```python
from build123d import *

# Parameters (mm, degrees)
SKETCH1_W           = 25.4
SKETCH1_H           = 25.4
BOSS_EXTRUDE1_DEPTH = 6.35


with BuildPart() as part:
    # Sketch1 → Boss-Extrude1 (new body)
    with BuildSketch(Plane.XY):
        with Locations((38.1, 241.3)):
            Rectangle(SKETCH1_W, SKETCH1_H)
        with Locations((88.9, 241.3)):
            Rectangle(SKETCH1_W, SKETCH1_H)
        with Locations((139.7, 241.3)):
            Rectangle(SKETCH1_W, SKETCH1_H)
        Polygon((0, 228.6), (0, 0), (177.8, 0), (177.8, 228.6), (152.4, 228.6), (127, 228.6), (116.0018, 228.6), (116.0018, 215.9), (117.1448, 215.9), (117.1448, 213.3092), (116.0018, 213.3092), (116.0018, 205.6892), (112.5982, 205.6892), (112.5982, 213.3092), (111.4552, 213.3092), (111.4552, 215.9), (112.5982, 215.9), (112.5982, 228.6), (101.6, 228.6), (76.2, 228.6), (65.2018, 228.6), (65.2018, 215.9), (66.3448, 215.9), (66.3448, 213.3092), (65.2018, 213.3092), (65.2018, 205.6892), (61.7982, 205.6892), (61.7982, 213.3092), (60.6552, 213.3092), (60.6552, 215.9), (61.7982, 215.9), (61.7982, 228.6), (50.8, 228.6), (25.4, 228.6), align=None)
    extrude(amount=BOSS_EXTRUDE1_DEPTH)


solid = part.part
```
The listing builds one solid part. Answer for the finished solid, in the listing's coordinates (mm). A direction names the side the tool comes from. Give positions to 0.01 mm unless a question says otherwise; leave off trailing zeros. Loops run counter-clockwise (first coordinate to the right, second up) from the corner with the lowest first, then second, coordinate; pieces in that order, holes last. Notation, with made-up numbers: M -4.75,-20.5 L 36.25,-20.5 A13 cw 36.25,-7.5 Z; hole C 50.25,71 d11. An arc over 180 degrees is marked long. One line per item, written item: value.
1. For faces 4 (the face through (13, 228.6, 3)), 5 (the face through (71, 228.6, 3)), 6 (the face through (152.4, 241, 3)), determine the directions among +Z, -Z, +X, -X, +Y, -Y from which every point of the face is accessible in a straight line to the end or side of a thin tool.
Found:
face 4: +Z, -Z, -X, +Y
face 5: +Z, -Z, +Y
face 6: +Z, -Z, +X, +Y
2. For a pull along X with two mould halves and no side action, classify faces 1 (the face through (88, 0, 3)), 2 (the face through (0, 116, 3)), 3 (the face through (61.798, 222, 3)) as pulls with the +X half, pulls with the -X half, needs draft (parallel to the pull), parting line crosses it, or undercut.
Found:
face 1: needs draft
face 2: pulls with the -X half
face 3: undercut
3. Section A-A on y = 210 is taken. Determine the outline of the cut face in (x, z).
Found:
outline: M 0,0 L 61.8,0 L 61.8,6.35 L 0,6.35 Z; M 65.2,0 L 112.6,0 L 112.6,6.35 L 65.2,6.35 Z; M 116,0 L 177.8,0 L 177.8,6.35 L 116,6.35 Z
4. Each of these flat-tipped pins is pushed along its axis until it touches: P1, Ø3, axis at x = 8, z = 2.5, coming from the +Y side; P2, Ø1.3, axis at y = 214, z = 2.5, coming from the -X side; P3, Ø1.9, axis at y = 236.5, z = 4, coming from the -X side; P4, Ø1, axis at x = 115, z = 4.5, coming from the +Y side. Where does it stop, or does it pass through?
Found:
P1: y = 228.6
P2: x = 0
P3: x = 25.4
P4: y = 205.69
5. Find the intervals of material crossed by probe 1 along Y at (x, z) = (112, 4); probe 2 along Y at (x, z) = (68, 4.5), in increasing order.
Found:
probe 1: 0 to 213.31, 215.9 to 228.6
probe 2: 0 to 228.6
6. Section B-B on x = 166.5 is taken. Determine the outline of the cut face in (y, z), plus the area to 3 significant figures.
Found:
outline: M 0,0 L 228.6,0 L 228.6,6.35 L 0,6.35 Z
area: 1,450 mm^2
